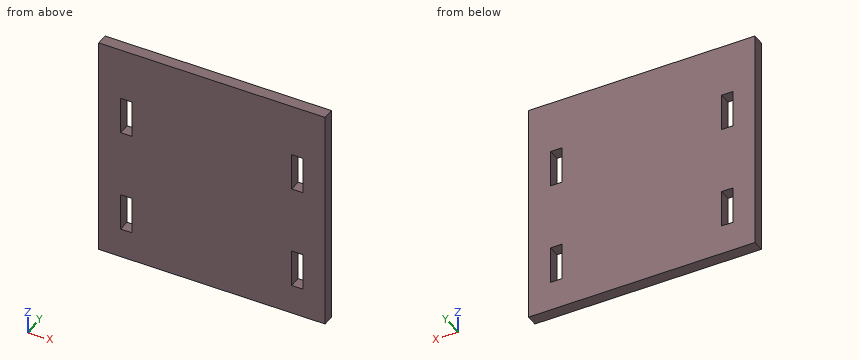
```python
from build123d import *

# Parameters (mm, degrees)
F0_W     = 19.1008
F0_H     = 63.5
F1_DEPTH = 19.3294


with BuildPart() as f1:
    # F0 (on Front) → F1 (new body)
    with BuildSketch(Plane.XZ):
        Polygon((263.06506, 395.92291), (-117.93494, 395.92291), (-118.136241, 14.92291), (263.06506, 14.787505), align=None)
        Polygon((-81.015004, 129.087942), (-61.914204, 129.087942), (-61.682431, 65.702861), (-81.04849, 65.709486), align=None, mode=Mode.SUBTRACT)
        with Locations((216.45606, 97.357456)):
            Rectangle(F0_W, F0_H, mode=Mode.SUBTRACT)
        Polygon((-80.956865, 243.503396), (-80.923315, 307.003359), (-61.822515, 307.003359), (-61.924184, 243.509798), align=None, mode=Mode.SUBTRACT)
        with Locations((216.45606, 275.27291)):
            Rectangle(F0_W, F0_H, mode=Mode.SUBTRACT)
    extrude(amount=F1_DEPTH)


solid = f1.part
```
Check sheet for the modelled part. Datum: model origin and axes. Units: mm. Give positions to 0.01 mm unless a question says otherwise; leave off trailing zeros. Write each loop counter-clockwise with the first axis right and the second up, starting at its lowest first coordinate (ties: lowest second). Pieces come first, ordered by that corner, then holes. Notation, with made-up numbers: (44, -16) - (79, -16) arc R26 cw to (79, 13) - close; hole circle Ø6 at (9.5, 0.25). An arc over 180 degrees is marked (long way). Answer as a JSON object with one key per item and string values. Group by question number.
1) Depth check by flat-ended pin: P1, Ø9.5, axis at y = -10.5, z = 276, coming from the -X side; P2, Ø10, axis at x = 180, y = -11.5, coming from the -Z side; P3, Ø5.5, axis at x = -71, y = -14, coming from the -Z side. Enter the tip coordinate at first touch or a pass-through.
2) Thickness scan on probe 1 along Z at (x, y) = (216.5, -18.25); probe 2 along X at (y, z) = (-2.5, 66); probe 3 along X at (y, z) = (-7, 93.5). Record the ranges inside material, lowest first. Write a range as from..to.
3) Sectioned sample at A-A (y = -10). Record the cut outline in (x, z) (1 decimal), then the cut area to 3 significant figures.
4) Sectioned sample at B-B (z = 265.5). Record the cut outline in (x, y), then the cut area to 3 significant figures.
Geometry results:
{
 "1": {"P1": "stops at x = -118", "P2": "stops at z = 14.82", "P3": "stops at z = 14.91"},
 "2": {"probe 1": "z = 14.8..65.61, 129.11..243.52, 307.02..395.92", "probe 2": "x = -118.11..-81.05, -61.68..206.91, 226.01..263.07", "probe 3": "x = -118.09..-81.03, -61.78..206.91, 226.01..263.07"},
 "3": {"outline": "(-118.1, 14.9) - (263.1, 14.8) - (263.1, 395.9) - (-117.9, 395.9) - close; hole (-81, 65.7) - (-61.7, 65.7) - (-61.9, 129.1) - (-81, 129.1) - close; hole (-81, 243.5) - (-61.9, 243.5) - (-61.8, 307) - (-80.9, 307) - close; hole (206.9, 65.6) - (226, 65.6) - (226, 129.1) - (206.9, 129.1) - close; hole (206.9, 243.5) - (226, 243.5) - (226, 307) - (206.9, 307) - close", "area": "140,000 mm^2"},
 "4": {"outline": "(-118, -19.33) - (-80.95, -19.33) - (-80.95, 0) - (-118, 0) - close; (-61.89, -19.33) - (206.91, -19.33) - (206.91, 0) - (-61.89, 0) - close; (226.01, -19.33) - (263.07, -19.33) - (263.07, 0) - (226.01, 0) - close", "area": "6,630 mm^2"}
}
